Build history of the part. All positions in model axes, mm. A direction names the side the tool comes from. Round coordinates to 2 decimals unless told otherwise and drop trailing zeros. Loops run counter-clockwise (first coordinate to the right, second up) from the corner with the lowest first, then second, coordinate; pieces in that order, holes last. Notation, with made-up numbers: (-9.5, 18.25) - (47.5, 18.25) arc R17 cw to (47.5, 23.25) - close; hole circle Ø3 at (16, 75). An arc over 180 degrees is marked (long way). Answer as CSV lines item,"result". Start each with the question number.
```python
from build123d import *

# Parameters (mm, degrees)
SKETCH1_W           = 75
SKETCH1_H           = 25
BOSS_EXTRUDE1_DEPTH = 5
SKETCH2_W           = 5
SKETCH2_H           = 15
BOSS_EXTRUDE3_DEPTH = 105
SKETCH3_R           = 5
CUT_EXTRUDE1_DEPTH  = 41
SKETCH4_R           = 5
CUT_EXTRUDE2_DEPTH  = 41


with BuildPart() as part:
    # Sketch1 → Boss-Extrude1 (new body)
    with BuildSketch(Plane(origin=(0, 0, 0), x_dir=(1, 0, 0), z_dir=(0, 1, 0))):
        with Locations((84.381711682, 3.75)):
            Rectangle(SKETCH1_W, SKETCH1_H)
    extrude(amount=BOSS_EXTRUDE1_DEPTH)

    # Sketch2 → Boss-Extrude3 (add)
    with BuildSketch(Plane(origin=(0, 5, 0), x_dir=(1, 0, 0), z_dir=(0, 1, 0))):
        with Locations((84.381711682, 3.75)):
            Rectangle(SKETCH2_W, SKETCH2_H)
    extrude(amount=BOSS_EXTRUDE3_DEPTH)

    # Sketch3 → Cut-Extrude1 (cut, through all)
    with BuildSketch(Plane.ZY.offset(-81.881711682)):
        with Locations((-3.75, 13)):
            Circle(SKETCH3_R)
    extrude(amount=-CUT_EXTRUDE1_DEPTH, mode=Mode.SUBTRACT)

    # Sketch4 → Cut-Extrude2 (cut, through all)
    with BuildSketch(Plane.ZY.offset(-81.881711682)):
        with Locations((-3.75, 99)):
            Circle(SKETCH4_R)
    extrude(amount=-CUT_EXTRUDE2_DEPTH, mode=Mode.SUBTRACT)


solid = part.part
```
Q1. Pin check, flat tips, straight feed: pin 1 Ø4 at (x, z) = (77.5, -7.5) entering from +Y; pin 2 Ø8 at (y, z) = (61, 4) entering from -X; pin 3 Ø12 at (y, z) = (18, 4.5) entering from +X. Stop position of each tip, or through.
Q2. Band-saw the part on C-C, the plane x = 59. List the corners of the cut face in (y, z).
Q3. Band-saw the part on A-A, the plane z = -3.75. List the corners of the cut face in (x, y), then the cut area to 3 significant figures.
Q4. Band-saw the part on D-D, the plane y = 21.5. List the corners of the cut face in (x, z).
Q5. Tool access for faces 1 (the flat face through (81.882, 57, -4)), 2 (the flat face through (86.882, 57, -4)), 3 (the flat face through (84, 57, -11.25)), 4 (the flat face through (84, 57, 3.75)): list every direction of +Z, -Z, +X, -X, +Y, -Y with a clear straight run to the whole face (end or side of a thin tool).
Q6. Two-plate mould, pull along Y, no slides. Class faces 5 (the flat face through (84, 2, -16.25)), 6 (the cylindrical face through (84.347, 13.22, -8.745)), 7 (the flat face through (84, 110, -4)), 8 (the cylindrical face through (84.35, 94.12, -4.83)): released by +Y, released by -Y, zero draft, split by the parting line, or undercut.
Q7. Wall check: probe 1 along Y at (x, z) = (85.2, -3.75); probe 2 along X at (y, z) = (49, -5); probe 3 along Y at (x, z) = (53.5, -2.5). Give the ranges that are in metal, low to high. Write a range as [from, to].
Q8. Band-saw the part on B-B, the plane y = 99. List the corners of the cut face in (x, z).
Reported:
1,pin 1,"stops at y = 5"
1,pin 2,"stops at x = 81.88"
1,pin 3,"stops at x = 86.88"
2,outline,"(0, -16.25) - (5, -16.25) - (5, 8.75) - (0, 8.75) - close"
3,outline,"(46.88, 0) - (121.88, 0) - (121.88, 5) - (86.88, 5) - (86.88, 8) - (81.88, 8) - (81.88, 5) - (46.88, 5) - close; (81.88, 18) - (86.88, 18) - (86.88, 94) - (81.88, 94) - close; (81.88, 104) - (86.88, 104) - (86.88, 110) - (81.88, 110) - close"
3,area,"800 mm2"
4,outline,"(81.88, -11.25) - (86.88, -11.25) - (86.88, 3.75) - (81.88, 3.75) - close"
5,face 1,"+Z, -Z, -X, +Y"
5,face 2,"+Z, -Z, +X, +Y"
5,face 3,"-Z, +X, -X, +Y"
5,face 4,"+Z, +X, -X, +Y"
6,face 5,"zero draft"
6,face 6,"undercut"
6,face 7,"released by +Y"
6,face 8,"undercut"
7,probe 1,"y = [0, 8], [18, 94], [104, 110]"
7,probe 2,"x = [81.88, 86.88]"
7,probe 3,"y = [0, 5]"
8,outline,"(81.88, -11.25) - (86.88, -11.25) - (86.88, -8.75) - (81.88, -8.75) - close; (81.88, 1.25) - (86.88, 1.25) - (86.88, 3.75) - (81.88, 3.75) - close"
